from build123d import *

# Parameters (mm, degrees)
F0_R            = 6.35
F0_R_2          = 2.38125
F1_DEPTH        = 4.7625
F3_DEPTH        = 4.7635
F3_COPIES_COUNT = 34


# Not quite as in the source:
# - a pattern or mirror of a feature is missing from the dataset's text; its kind, count and spacing are read off the source's solid


with BuildPart() as f1:
    # F0 (on Front) → F1 (new body)
    with BuildSketch(Plane.XZ):
        Circle(F0_R)
        Circle(F0_R_2, mode=Mode.SUBTRACT)
    extrude(amount=F1_DEPTH)

    # F2 (on Front) → F3 (cut, through all)
    with BuildSketch(Plane.XZ):
        with BuildLine():
            Line((-0.5859040826, 6.3229120195), (0, 5.969))
            Line((0, 5.969), (0.5859040826, 6.3229120195))
            ThreePointArc((0.5859040826, 6.3229120195), (0, 6.4661394577), (-0.5859040826, 6.3229120195))
        make_face()
    f3 = extrude(amount=F3_DEPTH, mode=Mode.SUBTRACT)

    # F3_copies: F3 ×34 about axis
    f3_copies_axis = Axis((0, 0, 0), (0, 1, 0))
    for i in range(1, F3_COPIES_COUNT):
        add(f3.rotate(f3_copies_axis, i * 360 / F3_COPIES_COUNT), mode=Mode.SUBTRACT)


solid = f1.part
Design review of the part built by this model. Coordinates are the model's own, in mm. Coordinates: 2 decimals unless noted, no trailing zeros. Loops run counter-clockwise (first coordinate to the right, second up) from the corner with the lowest first, then second, coordinate; pieces in that order, holes last. Notation, with made-up numbers: M 81.5,20.25 L 119.5,20.25 A17 ccw 119.5,51.25 Z; hole C 20.25,-15 d9. An arc over 180 degrees is marked long. Use one line per item in the form item = value.
(1) Consider section C-C (z = -4). Write out the cut boundary in (x, y), and give its area (3 significant figures).
Return value:
outline = M -4.72,-4.76 L 4.72,-4.76 L 4.72,0 L -4.72,0 Z
area = 45.0 mm2
(2) For line 1 along Z through (x, y) = (-0.75, -2.25); line 2 along Z through (x, y) = (2, -1.5); line 3 along X through (y, z) = (-0.7, 0.5), list the stretches that pass through material, from the lowest coordinate up. Write a range as from..to.
Return value:
line_1 = -6.18..-2.26, 2.26..6.18
line_2 = -5.77..-1.29, 1.29..5.77
line_3 = -5.98..-2.33, 2.33..5.98
(3) Clearance check with flat-ended pins moving along their axes: P1, Ø1.5, axis at y = -2.5, z = -1, coming from the +X side; P2, Ø1, axis at y = -4.5, z = 3.5, coming from the +X side; P3, Ø4, axis at x = 0, z = 0, coming from the +Y side; P4, Ø1, axis at y = -1.5, z = -2.5, coming from the -X side. State where each tip first meets the part, or that it passes through.
Return value:
P1 = 6.24
P2 = 5.4
P3 = through
P4 = -5.92
(4) Consider section B-B (x = 3.5). Write out the cut boundary in (y, z), and give its area (3 significant figures).
Return value:
outline = M -4.76,-5.07 L 0,-5.07 L 0,5.07 L -4.76,5.07 Z
area = 48.3 mm2
(5) Draft analysis for pull direction X (two halves, no side actions). For faces 1 (the face through (0, -4.762, -3)), 2 (the face through (-1.89, -2.35, -1.45)), state which applies: pulls with the +X half, pulls with the -X half, needs draft (parallel to the pull), parting line crosses it, or undercut.
Return value:
face_1 = needs draft
face_2 = undercut
(6) Consider section A-A (z = 1). Write out the cut boundary in (x, y).
Return value:
outline = M -6.16,-4.76 L -2.16,-4.76 L -2.16,0 L -6.16,0 Z; M 2.16,-4.76 L 6.16,-4.76 L 6.16,0 L 2.16,0 Z
